Can you work these out from the model? Positions are in its coordinate system, mm. Face numbers are marked on the shaded views. Round coordinates to 2 decimals unless told otherwise and drop trailing zeros. Write each loop counter-clockwise with the first axis right and the second up, starting at its lowest first coordinate (ties: lowest second). Pieces come first, ordered by that corner, then holes. Notation, with made-up numbers: (46.5, 12.5) -> (61.5, 12.5) arc R21 cw to (61.5, 24.5) -> close; hole circle Ø10 at (82.25, 64.25). An arc over 180 degrees is marked (long way). Use CSV: the item, a comma, the result in double quotes.
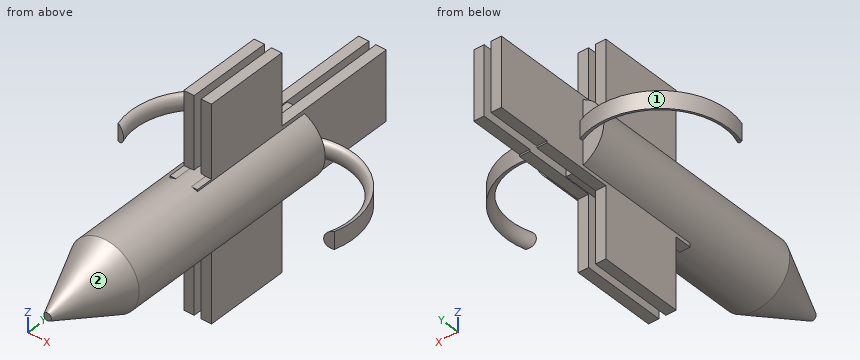
```python
from build123d import *

# Parameters (mm, degrees)
F0_W      = 24.6273766255
F0_H      = 152.4
F3_R      = 25.4
F4_DEPTH  = 82.55
F8_W      = 62.4961581021
F8_H      = 152.4
F9_DEPTH  = 7.62
F11_W     = 127
F11_H     = 50.8
F12_DEPTH = 7.62
F13_W     = 152.4
F13_H     = 76.2
F14_DEPTH = 7.62
F15_R     = 25.4
F16_DEPTH = 50.8
F16_TAPER = 24
F17_DEPTH = 25.4


with BuildPart() as f1:
    # F0 (on Top) → F1 (revolve)
    with BuildSketch(Plane.XY):
        with Locations((1.4390293509, 0)):
            Rectangle(F0_W, F0_H)
    revolve(axis=Axis((13.7527176636, 0, 0), (0, -1, 0)))


with BuildPart() as f4:
    # F3 (on Front) → F4 (new body, symmetric)
    with BuildSketch(Plane.XZ):
        Circle(F3_R)
    extrude(amount=F4_DEPTH, both=True)

    # F8 (on offset) → F9 (join)
    with BuildSketch(Plane.YZ.offset(2.54)):
        with Locations((31.2480790511, 2.0054676748)):
            Rectangle(F8_W, F8_H)
    extrude(amount=F9_DEPTH)

    # F10: F4 across plane


with BuildPart() as f4_1:
    add(f4.part)
    add(f4.part.mirror(Plane.XY))

    # F11 (on offset) → F12 (join)
    with BuildSketch(Plane.YZ.offset(2.54)):
        with Locations((51.0253053619, -0.6605200469)):
            Rectangle(F11_W, F11_H)
    extrude(amount=F12_DEPTH)

    # F13 (on offset) → F14 (join)
    with BuildSketch(Plane.YZ.offset(2.54)):
        with Locations((79.006247285, 13.3819643736)):
            Rectangle(F13_W, F13_H)
    extrude(amount=F14_DEPTH)

    # F15 (on face) → F16 (join)
    with BuildSketch(Plane.XZ.offset(82.55)):
        Circle(F15_R)
    extrude(amount=F16_DEPTH, taper=F16_TAPER)

    # F17 (cut): faces of the model
    f17_faces = [f4_1.faces().sort_by_distance(p)[0] for p in [
        (6.35, 108.8512026936, 51.4819643736),
        (6.35, 88.510731732, -26.0605200469),
    ]]
    extrude(f17_faces, amount=-F17_DEPTH, dir=(0, 0, 1), mode=Mode.SUBTRACT)

    # F20: sweep along a path in F18
    with BuildLine(Plane.XY) as f20_path:
        ThreePointArc((79.5428454876, 25.338916108), (15.8456347969, 87.7762718464), (0, 0))
    # F19 (on Right) → F20 (sweep)
    with BuildSketch(Plane.YZ):
        with BuildLine():
            ThreePointArc((0, -6.35), (6.35, 0), (0, 6.35))
            Line((0, 6.35), (0, -6.35))
        make_face()
    sweep(path=f20_path.line)

    # F21: F4 across plane


with BuildPart() as f4_2:
    add(f4_1.part)
    add(f4_1.part.mirror(Plane.YZ))


solid = f4_2.part
```
Q1. Suppose I cut it at B-B (y = -28.5). Write out the boundary of the cut face in (x, z), and give its area (3 significant figures).
Resolved:
outline,"circle Ø50.8 at (0, 0)"
area,"2,030 mm^2"
Q2. Please list where these lines run through material, in increasing order: probe 1 along X at (y, z) = (3, 65); probe 2 along Y at (x, z) = (-8.5, 55); probe 3 along Z at (x, y) = (-6, 97).
Resolved:
probe 1,"x = -10.16 to -2.54, 2.54 to 10.16"
probe 2,"y = 0 to 62.5"
probe 3,"z = -26.06 to 26.08"
Q3. Suppose I cut it at A-A (z = -38.5). Write out the boundary of the cut face in (x, y), and give its area (3 significant figures).
Resolved:
outline,"(-10.16, 0) -> (-2.54, 0) -> (-2.54, 62.5) -> (-10.16, 62.5) -> close; (2.54, 0) -> (10.16, 0) -> (10.16, 62.5) -> (2.54, 62.5) -> close"
area,"952 mm^2"
Q4. Suppose I cut it at C-C (y = 47). Count the separate pieces of the cut face and the enclosed holes in it, and give its area (3 significant figures).
Resolved:
separate pieces,"3"
enclosed holes,"0"
area,"3,760 mm^2"
Q5. Will these pins go through, and if not, where does the flat tip stop? P1, Ø3, axis at x = -8, z = -28, coming from the -Y side; P2, Ø6, axis at x = -5, z = -44, coming from the +Y side; P3, Ø2.5, axis at x = 4.5, y = 87.5, coming from the -Z side; P4, Ø10, axis at x = -44, z = 15, coming from the +Y side.
Resolved:
P1,"stops at y = 0"
P2,"stops at y = 62.5"
P3,"stops at z = -26.06"
P4,"passes through"
Q6. Suppose I cut it at D-D (y = -101). Write out the boundary of the cut face in (x, z), and give its area (3 significant figures).
Resolved:
outline,"circle Ø34.37 at (0, 0)"
area,"928 mm^2"
Q7. If we mould it in two halves opening along X, with no side actions, what happens to the marked faces 1 and 2? For each: released by +X, released by -X, zero draft, split by the parting line, or undercut.
Resolved:
face 1,"undercut"
face 2,"split by the parting line"
